```python
from build123d import *

# Parameters (mm, degrees)
F0_R     = 55.5
F1_DEPTH = 5
F2_R     = 3


with BuildPart() as f1:
    # F0 (on Top) → F1 (new body)
    with BuildSketch(Plane.XY):
        Circle(F0_R)
        Polygon((-43.6709144021, -28.8896496715), (-46.4835835158, -23.3083064231), (-49.2962526295, -17.7269631746), (-36.3475362931, -11.2015708309), (-30.7221980657, -22.3642573278), align=None, mode=Mode.SUBTRACT)
        with BuildLine():
            ThreePointArc((-25.9631257504, -24.5759761), (-32.2743582607, -15.3762251173), (-35.4424777104, -4.6790248716))
            Line((-35.4424777104, -4.6790248716), (-38.2146140403, -4.6790248716))
            ThreePointArc((-38.2146140403, -4.6790248716), (-17.8953589694, 34.0882109733), (25.553195754, 28.797294782))
            Line((25.553195754, 28.797294782), (23.8329245146, 26.6468423848))
            ThreePointArc((23.8329245146, 26.6468423848), (31.5030749277, 16.9002594685), (35.381527976, 5.1195681537))
            Line((35.381527976, 5.1195681537), (38.1580924827, 5.1195681537))
            ThreePointArc((38.1580924827, 5.1195681537), (16.7555959393, -34.6626600929), (-27.7152221959, -26.7229575203))
            Line((-27.7152221959, -26.7229575203), (-25.9631257504, -24.5759761))
        make_face(mode=Mode.SUBTRACT)
        Polygon((43.5800816552, 29.0698943851), (46.3897934183, 23.4944195798), (46.3927507689, 23.4885511366), (47.6104286529, 21.0722419435), (49.2024625319, 17.9130763314), (36.2537461955, 11.3876839877), (30.6313653188, 22.5445020413), align=None, mode=Mode.SUBTRACT)
    extrude(amount=F1_DEPTH)

    # F2
    f2_edges = [f1.edges().sort_by_distance(p)[0] for p in [
        (-36.347536, -11.201571, 2.5),
        (-49.296253, -17.726963, 2.5),
        (-30.722198, -22.364257, 2.5),
        (-43.670914, -28.88965, 2.5),
        (36.253746, 11.387684, 2.5),
        (30.631365, 22.544502, 2.5),
        (43.580082, 29.069894, 2.5),
        (49.202463, 17.913076, 2.5),
    ]]
    fillet(f2_edges, radius=F2_R)


solid = f1.part
```
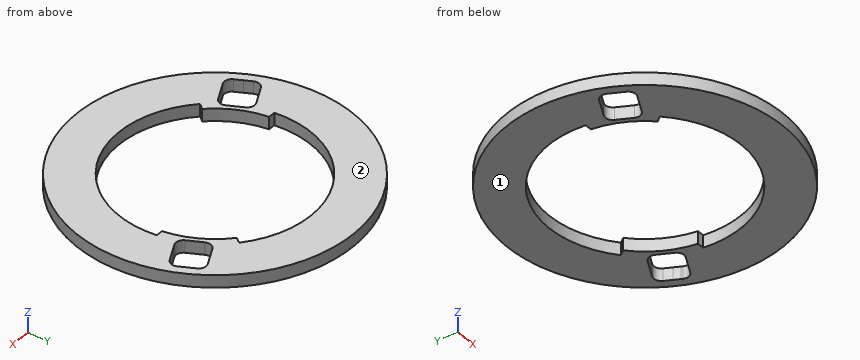
Can you work these out from the model? Positions are in its coordinate system, mm. Face numbers are marked on the shaded views. Coordinates: 2 decimals unless noted, no trailing zeros. Loops run counter-clockwise (first coordinate to the right, second up) from the corner with the lowest first, then second, coordinate; pieces in that order, holes last.
Item 1: Please list where these lines run through material, in increasing order: L1, parallel to Y at x = 33, z = 1.95; L2, parallel to Y at x = -7, z = 3.55; L3, parallel to X at y = -17.5, z = 0.85.
Answers below:
L1: y = -44.62 to -19.83, 13.75 to 17.84, 23.71 to 44.62
L2: y = -55.06 to -37.86, 37.86 to 55.06
L3: x = -52.67 to -47.83, -33.17 to -31.17, 34.29 to 52.67
Item 2: I'm going to push flat-ended pins straight in: pin 1 (1.4 mm diameter, centred on x = -37.5, z = 1.5, fed in from +Y); pin 2 (2 mm diameter, centred on x = 36.5, z = 3, fed in from -Y); pin 3 (1.5 mm diameter, centred on x = 26.5, z = 3, fed in from +Y). Where does each tip first touch, or does it pass through?
Answers below:
pin 1: stops at y = 41.55
pin 2: stops at y = -42.66
pin 3: stops at y = 49.16
Item 3: Suppose I cut it at B-B (z = 2.2). Please give me the cut outline in (x, y).
Answers below:
outline: circle Ø111 at (0, 0); hole (-47.95, -20.41) - (-45.02, -26.21) arc R3 ccw to (-40.99, -27.54) - (-33.4, -23.71) arc R3 ccw to (-32.07, -19.69) - (-35, -13.88) arc R3 ccw to (-39.03, -12.55) - (-46.62, -16.38) arc R3 ccw to start; hole (-38.21, -4.68) - (-35.44, -4.68) arc R35.75 ccw to (-25.96, -24.58) - (-27.72, -26.72) arc R38.5 ccw to (38.16, 5.12) - (35.38, 5.12) arc R35.75 ccw to (23.83, 26.65) - (25.55, 28.8) arc R38.5 ccw to start; hole (31.98, 19.87) - (34.9, 14.07) arc R3 ccw to (38.93, 12.74) - (46.52, 16.56) arc R3 ccw to (47.85, 20.59) - (44.93, 26.39) arc R3 ccw to (40.9, 27.72) - (33.31, 23.89) arc R3 ccw to start
Item 4: Suppose I cut it at A-A (y = 0). Please give me the cut outline in (x, z), then the cut area to 3 significant figures.
Answers below:
outline: (-55.5, 0) - (-38.5, 0) - (-38.5, 5) - (-55.5, 5) - close; (38.5, 0) - (55.5, 0) - (55.5, 5) - (38.5, 5) - close
area: 170 mm2
Item 5: If we mould it in two halves opening along Z, with no side actions, what happens to the marked faces 1 and 2? For each: released by +Z, released by -Z, zero draft, split by the parting line, or undercut.
Answers below:
face 1: released by -Z
face 2: released by +Z
Item 6: Suppose I cut it at D-D (y = -18). Please give me the cut outline in (x, z), then the cut area to 3 significant figures.
Answers below:
outline: (-52.5, 0) - (-48.08, 0) - (-48.08, 5) - (-52.5, 5) - close; (-32.92, 0) - (-30.89, 0) - (-30.89, 5) - (-32.92, 5) - close; (34.03, 0) - (52.5, 0) - (52.5, 5) - (34.03, 5) - close
area: 125 mm2
